Work out the finished part from the listing and answer in its coordinate system (mm). A direction names the side the tool comes from. Round coordinates to 2 decimals unless told otherwise and drop trailing zeros. Loops run counter-clockwise (first coordinate to the right, second up) from the corner with the lowest first, then second, coordinate; pieces in that order, holes last. Notation, with made-up numbers: (-35, -5) - (11, -5) arc R18 ccw to (11, 15) - close; hole circle Ø11 at (80.25, -31). An arc over 180 degrees is marked (long way). Answer as CSV lines item,"result". Start each with the question number.
Q1. Section A-A on y = 4.75 is taken. Write down the section's boundary in (x, z), then the cut area to 3 significant figures.
Q2. Straight lines are drawn through the part: L1, parallel to Z at x = 12.5, y = 1.25; L2, parallel to X at y = 4.75, z = 28; L3, parallel to Y at x = 14, z = 33.5. For each, find the intervals that lie inside material, in ascending order. Write a range as [from, to].
Q3. The mould has two halves that part along X. Classify faces 1 (the face through (0, 1, 18)), 2 (the face through (7, 0, 18)), 3 (the face through (1.838, 2.507, 7.384)), 4 (the face through (15.84, 6.44, 29.92)): +X half, -X half, draft (parallel to the pull), parting line (faces both ways), or undercut.
Q4. Section C-C on x = 4.5 is taken. Write down the section's boundary in (y, z).
Q5. Each of these flat-tipped pins is pushed along its axis until it touches: pin 1 Ø5 at (x, z) = (6.5, 23.5) entering from +Y; pin 2 Ø3.5 at (x, z) = (4.5, 6) entering from +Y; pin 3 Ø1.5 at (y, z) = (1.5, 20.5) entering from +X. Where does it stop, or does it pass through?
Q6. Section D-D on x = 14.5 is taken. Write down the section's boundary in (y, z), then the cut area to 3 significant figures.
Q7. For faces 5 (the face through (3, 2, 31)), 6 (the face through (9.058, 1, 18)), 7 (the face through (4.57, 1.01, 28.4)), determine the directions among +Z, -Z, +X, -X, +Y, -Y from which every point of the face is accessible in a straight line to the end or side of a thin tool.
Q8. Section B-B on z = 30 is taken. Write down the section's boundary in (x, y), then the cut area to 3 significant figures.
```python
from build123d import *

# Parameters (mm, degrees)
SKETCH_1_W          = 14
SKETCH_1_H          = 36
EXTRUDE_1_DEPTH     = 3
SKETCH_2_R          = 4.75
EXTRUDE_2_DEPTH     = 12
EXTRUDE_START       = -12
SKETCH_3_R          = 4.75
EXTRUDE_3_DEPTH     = 12
SKETCH_4_R          = 2.5
CUT_EXTRUDE_1_DEPTH = 51
SKETCH_5_W          = 8.893722196
SKETCH_5_H          = 10.697157082
CUT_EXTRUDE_2_DEPTH = 12
SKETCH_6_R          = 1.6
CUT_EXTRUDE_3_DEPTH = 10
SKETCH_7_R          = 3
CUT_EXTRUDE_4_DEPTH = 1


with BuildPart() as part:
    # 草图1 → 凸台-拉伸1 (new body)
    with BuildSketch(Plane(origin=(0, 0, 0), x_dir=(1, 0, 0), z_dir=(0, 1, 0))):
        with Locations((7, -18)):
            Rectangle(SKETCH_1_W, SKETCH_1_H)
    extrude(amount=EXTRUDE_1_DEPTH)

    # 草图2 → 凸台-拉伸2 (add)
    with BuildSketch(Plane(origin=(0, 0, 0), x_dir=(-1, 0, 0), z_dir=(0, 0, -1))):
        with Locations((-14, 4.75)):
            Circle(SKETCH_2_R)
    extrude(amount=-EXTRUDE_2_DEPTH)

    # 草图3 → 凸台-拉伸3 (add)
    with BuildSketch(Plane.XY.offset(36).offset(EXTRUDE_START)):
        with Locations((14, 4.75)):
            Circle(SKETCH_3_R)
    extrude(amount=EXTRUDE_3_DEPTH)

    # 草图4 → 切除-拉伸1 (cut)
    with BuildSketch(Plane(origin=(0, 0, 0), x_dir=(-1, 0, 0), z_dir=(0, 0, -1))):
        with Locations((-14, 4.75)):
            Circle(SKETCH_4_R)
    extrude(amount=-CUT_EXTRUDE_1_DEPTH, mode=Mode.SUBTRACT)

    # 草图5 → 切除-拉伸2 (cut)
    with BuildSketch(Plane(origin=(0, 0, 24), x_dir=(-1, 0, 0), z_dir=(0, 0, -1))):
        with Locations((-13.504665101, 2.655560542)):
            Rectangle(SKETCH_5_W, SKETCH_5_H)
    extrude(amount=CUT_EXTRUDE_2_DEPTH, mode=Mode.SUBTRACT)

    # 草图6 → 切除-拉伸3 (cut)
    with BuildSketch(Plane(origin=(0, 3, 0), x_dir=(1, 0, 0), z_dir=(0, 1, 0))):
        with Locations(Location((4.5, -6, 0), (0, 0, 270))):
            Circle(SKETCH_6_R)
        with Locations(Location((4.5, -30, 0), (0, 0, 270))):
            Circle(SKETCH_6_R)
    extrude(amount=-CUT_EXTRUDE_3_DEPTH, mode=Mode.SUBTRACT)

    # 草图7 → 切除-拉伸4 (cut)
    with BuildSketch(Plane(origin=(0, 3, 0), x_dir=(1, 0, 0), z_dir=(0, 1, 0))):
        with Locations(Location((4.5, -6, 0), (0, 0, 270))):
            Circle(SKETCH_7_R)
        with Locations(Location((4.5, -30, 0), (0, 0, 270))):
            Circle(SKETCH_7_R)
    extrude(amount=-CUT_EXTRUDE_4_DEPTH, mode=Mode.SUBTRACT)


solid = part.part
```
Findings:
1,outline,"(9.25, 0) - (11.5, 0) - (11.5, 12) - (9.25, 12) - close; (9.25, 24) - (11.5, 24) - (11.5, 36) - (9.25, 36) - close; (16.5, 0) - (18.75, 0) - (18.75, 12) - (16.5, 12) - close; (16.5, 24) - (18.75, 24) - (18.75, 36) - (16.5, 36) - close"
1,area,"108 mm^2"
2,L1,"z = [0, 12], [24, 36]"
2,L2,"x = [9.25, 11.5], [16.5, 18.75]"
2,L3,"y = [0, 2.25], [7.25, 9.5]"
3,face 1,"-X half"
3,face 2,"draft"
3,face 3,"undercut"
3,face 4,"undercut"
4,outline,"(0, 0) - (3, 0) - (3, 3) - (2, 3) - (2, 4.4) - (0, 4.4) - close; (0, 7.6) - (2, 7.6) - (2, 9) - (3, 9) - (3, 27) - (2, 27) - (2, 28.4) - (0, 28.4) - close; (0, 31.6) - (2, 31.6) - (2, 33) - (3, 33) - (3, 36) - (0, 36) - close"
5,pin 1,"stops at y = 3"
5,pin 2,"stops at y = 2"
5,pin 3,"stops at x = 9.06"
6,outline,"(0.03, 0) - (2.3, 0) - (2.3, 12) - (0.03, 12) - close; (0.03, 24) - (2.3, 24) - (2.3, 36) - (0.03, 36) - close; (7.2, 0) - (9.47, 0) - (9.47, 12) - (7.2, 12) - close; (7.2, 24) - (9.47, 24) - (9.47, 36) - (7.2, 36) - close"
6,area,"109 mm^2"
7,face 5,"+Y"
7,face 6,"+X, +Y, -Y"
7,face 7,"+Y, -Y"
8,outline,"(0, 0) - (2.9, 0) - (2.9, 2) - (1.5, 2) - (1.5, 3) - (0, 3) - close; (6.1, 0) - (14, 0) arc R4.75 ccw (long way) to (9.58, 3) - (7.5, 3) - (7.5, 2) - (6.1, 2) - close; hole circle Ø5 at (14, 4.75)"
8,area,"71.2 mm^2"
